Autodesk Fusion 360 part; units mm, degrees
sketch "Sketch1" plane through (0, 0, 0) normal (0, 1, 0) x (1, 0, 0)
  circle A0 centre (0, 0) radius 5
  dimension "d1" = 10
extrude "Extrude1" add sketch "Sketch1" along normal blind 70 makes body 1
copy_body "Body->Comp1" bodies 1 removing the originals makes body 2 in component "Component"
component "Component" placed x (1, 0, 0) y (0, 1, 0) z (0, 0, 1) at (0, 0, 0)
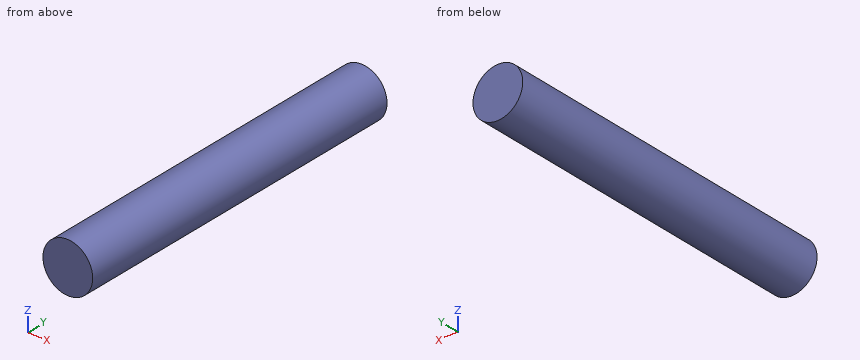
Can you work these out from the model? Positions are in its coordinate system, mm. Give positions to 0.01 mm unless a question says otherwise; leave off trailing zeros. Order: outer loops, then holes, each group sorted by start corner. A loop starts at its lowest first (then second) coordinate and runs counter-clockwise, first axis right, second up. Notation, with made-up numbers: M 77,12 L 122,12 A21 ccw 122,34 Z; hole C -9,13 d10. An arc over 180 degrees is marked long. One line per item, written item: value.
1) For P1, Ø3, axis at x = -2, y = 10, coming from the +Z side; P2, Ø3, axis at x = -3.5, y = 36, coming from the -Z side; P3, Ø2, axis at y = 58.5, z = -1.5, coming from the +X side, each with a flat end and sliding along its axis, tell me the tip position at first contact or that it passes through.
Answer sheet:
P1: stops at z = 4.97
P2: stops at z = -4.58
P3: stops at x = 4.97
2) Please list where these lines run through material, in increasing order: line 1 along X through (y, z) = (23, -2.5); line 2 along X through (y, z) = (39.5, -3); line 3 along Z through (x, y) = (1.5, 54).
Answer sheet:
line 1: x = -4.33 to 4.33
line 2: x = -4 to 4
line 3: z = -4.77 to 4.77
3) I want a section at A-A, the plane y = 31.5. List the corners of the cut face in (x, z) for me, plus the area to 3 significant figures.
Answer sheet:
outline: C 0,0 d10
area: 78.5 mm^2
4) I want a section at C-C, the plane z = 3.25. List the corners of the cut face in (x, y) for me, plus the area to 3 significant figures.
Answer sheet:
outline: M -3.8,0 L 3.8,0 L 3.8,70 L -3.8,70 Z
area: 532 mm^2
5) I want a section at B-B, the plane x = 1. List the corners of the cut face in (y, z) for me, plus the area to 3 significant figures.
Answer sheet:
outline: M 0,-4.9 L 70,-4.9 L 70,4.9 L 0,4.9 Z
area: 686 mm^2
